For this review, use the dimensioned drawing (mm, ordinates from the lowest corner) and the shaded views. Coordinates: 2 decimals unless noted, no trailing zeros. Loops run counter-clockwise (first coordinate to the right, second up) from the corner with the lowest first, then second, coordinate; pieces in that order, holes last. Notation, with made-up numbers: M 39.25,71 L 80.25,71 A16 cw 80.25,91 Z; hole C 59.25,89.5 d7. An arc over 180 degrees is marked long. One line per item, written item: value.
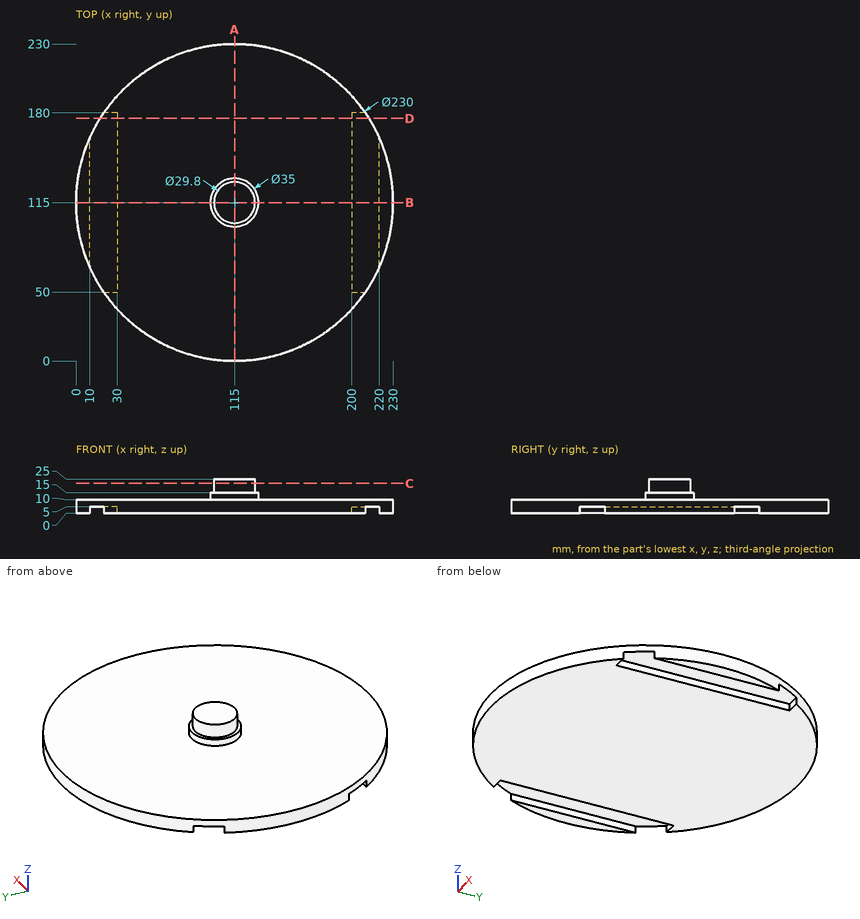
(1) We need section B-B on y = 115. State the section outline as (x, z) points.
Reply:
outline: M 0,0 L 10,0 L 10,5 L 30,5 L 30,0 L 200,0 L 200,5 L 220,5 L 220,0 L 230,0 L 230,10 L 132.5,10 L 132.5,15 L 129.9,15 L 129.9,25 L 100.1,25 L 100.1,15 L 97.5,15 L 97.5,10 L 0,10 Z
(2) To check wall thickness, follow line 1 along X through (y, z) = (155.5, 2); line 2 along Z through (x, y) = (197, 158.5); line 3 along X through (y, z) = (121, 1.5). State the ranges of each line that lie inside material, in increasing order. Write a range as [from, to].
Reply:
line 1: x = [7.37, 10], [30, 200], [220, 222.63]
line 2: z = [0, 10]
line 3: x = [0.16, 10], [30, 200], [220, 229.84]
(3) We need section C-C on z = 21.75. State the section outline as (x, y) points.
Reply:
outline: C 115,115 d29.8
(4) We need section D-D on y = 176. State the section outline as (x, z) points.
Reply:
outline: M 17.51,5 L 30,5 L 30,0 L 200,0 L 200,5 L 212.49,5 L 212.49,10 L 17.51,10 Z
(5) Insertion check: pin 1 (5 mm diameter, centred on x = 154, z = 10, fed in from -Y); pin 2 (4 mm diameter, centred on x = 25, z = 1.5, fed in from +Y); pin 3 (10 mm diameter, centred on x = 22, y = 100.5, fed in from -Z). Each pin has a flat end and moves straight along its axis. Give the tip position at first contact, or say it passes through.
Reply:
pin 1: stops at y = 5.95
pin 2: stops at y = 189.03
pin 3: stops at z = 5
(6) We need section A-A on x = 115. State the section outline as (y, z) points.
Reply:
outline: M 0,0 L 230,0 L 230,10 L 132.5,10 L 132.5,15 L 129.9,15 L 129.9,25 L 100.1,25 L 100.1,15 L 97.5,15 L 97.5,10 L 0,10 Z
